from build123d import *

# Parameters (mm, degrees)
SKETCH1_W               = 48
SKETCH1_H               = 45
BOSS_EXTRUDE1_DEPTH     = 3
BOSS_EXTRUDE2_DEPTH     = 37
SKETCH3_W               = 3
SKETCH3_H               = 40
BOSS_EXTRUDE3_DEPTH     = 30
BOSS_EXTRUDE4_DEPTH     = 3
FILLET1_R               = 10
FILLET2_R               = 5
CHAMFER1_SIZE           = 2
SKETCH5_R               = 1.75
SKETCH5_R_2             = 12.5
CUT_EXTRUDE1_DEPTH      = 91.65064234
RIB2_REACH              = 82.792
SKETCH6_WALL_W          = 183.583291708
SKETCH6_WALL_H          = 5
LPATTERN2_COUNT         = 2
LPATTERN2_PITCH         = 15
MIRROR1_COPY_1_REACH    = 82.792
MIRROR1_COPY_1_SKETCH_W = 183.583291708
MIRROR1_COPY_1_SKETCH_H = 5
SKETCH7_R               = 1.75
CUT_EXTRUDE2_DEPTH      = 97.982157929


with BuildPart() as part:
    # Sketch1 → Boss-Extrude1 (new body)
    with BuildSketch(Plane(origin=(0, 0, 0), x_dir=(1, 0, 0), z_dir=(0, 1, 0))):
        with Locations((0, -1.5)):
            Rectangle(SKETCH1_W, SKETCH1_H)
    extrude(amount=BOSS_EXTRUDE1_DEPTH)

    # Sketch2 → Boss-Extrude2 (add)
    with BuildSketch(Plane.XZ):
        Polygon((-21, 21), (21, 21), (21, -21), (24, -21), (24, 24), (-24, 24), (-24, -21), (-21, -21), align=None)
    extrude(amount=BOSS_EXTRUDE2_DEPTH)

    # Sketch3 → Boss-Extrude3 (add)
    with BuildSketch(Plane(origin=(24, 0, 0), x_dir=(0, 0, -1), z_dir=(1, 0, 0))):
        with Locations((19.5, -17)):
            Rectangle(SKETCH3_W, SKETCH3_H)
    extrude(amount=BOSS_EXTRUDE3_DEPTH)

    # Sketch4 → Boss-Extrude4 (add)
    with BuildSketch(Plane(origin=(0, 0, -21), x_dir=(-1, 0, 0), z_dir=(0, 0, -1))):
        Polygon((24, 3), (65.213203436, -38.213203436), (45.213203436, -58.213203436), (24, -37), align=None)
    extrude(amount=-BOSS_EXTRUDE4_DEPTH)

    # Fillet1
    fillet1_edges = [part.edges().sort_by_distance(p)[0] for p in [
        (24, -17, -18),
        (-24, -17, -18),
    ]]
    fillet(fillet1_edges, radius=FILLET1_R)

    # Fillet2
    fillet2_edges = [part.edges().sort_by_distance(p)[0] for p in [
        (21, -18.5, -21),
        (-21, -18.5, -21),
    ]]
    fillet(fillet2_edges, radius=FILLET2_R)

    # Chamfer1
    chamfer1_edges = [part.edges().sort_by_distance(p)[0] for p in [
        (24, -17, 24),
        (-24, -17, 24),
    ]]
    chamfer(chamfer1_edges, length=CHAMFER1_SIZE)

    # Sketch5 → Cut-Extrude1 (cut, through all)
    with BuildSketch(Plane.XZ):
        with Locations(Location((-15.5, 15.5, 0), (0, 0, 270))):
            Circle(SKETCH5_R)
        with Locations(Location((15.5, 15.5, 0), (0, 0, 270))):
            Circle(SKETCH5_R)
        with Locations(Location((15.5, -15.5, 0), (0, 0, 270))):
            Circle(SKETCH5_R)
        with Locations(Location((-15.5, -15.5, 0), (0, 0, 270))):
            Circle(SKETCH5_R)
        with Locations(Location((0, 0, 0), (0, 0, 270))):
            Circle(SKETCH5_R_2)
    extrude(amount=-CUT_EXTRUDE1_DEPTH, mode=Mode.SUBTRACT)

    # Sketch6 wall → Rib2 (add, up to next)
    with BuildSketch(Plane(origin=(-31.071067812, -17, -10.928932188), x_dir=(-0.707106781187, 0, -0.707106781187), z_dir=(-0.707106781187, 0, 0.707106781187)), mode=Mode.PRIVATE) as rib2_sk1:
        Rectangle(SKETCH6_WALL_W, SKETCH6_WALL_H)
    rib2_tool1 = extrude(rib2_sk1.sketch, amount=-RIB2_REACH, mode=Mode.PRIVATE) - part.part
    rib2 = rib2_tool1.solids().sort_by_distance((-31.071067812, -17, -10.928932188))[0]
    add(rib2)

    # LPattern2: Rib2 ×2
    with Locations(*[(0, -i * LPATTERN2_PITCH, 0) for i in range(1, LPATTERN2_COUNT)]):
        add(rib2)

    # Mirror1: Rib2 across plane
    add(rib2.mirror(Plane(origin=(0, 0, 0), x_dir=(0, 0, 1), z_dir=(1, 0, 0))))

    # Mirror1 copy 1 sketch → Mirror1 copy 1 (add, up to next)
    with BuildSketch(Plane(origin=(31.071067812, -32, -10.928932188), x_dir=(0.707106781187, 0, -0.707106781187), z_dir=(0.707106781187, 0, 0.707106781187)), mode=Mode.PRIVATE) as mirror1_copy_1_sk1:
        Rectangle(MIRROR1_COPY_1_SKETCH_W, MIRROR1_COPY_1_SKETCH_H)
    mirror1_copy_1_tool1 = extrude(mirror1_copy_1_sk1.sketch, amount=-MIRROR1_COPY_1_REACH, mode=Mode.PRIVATE) - part.part
    add(mirror1_copy_1_tool1.solids().sort_by_distance((31.071067812, -32, -10.928932188))[0])

    # Sketch7 → Cut-Extrude2 (cut, through all)
    with BuildSketch(Plane.XY.offset(-18)):
        with Locations((44, -7)):
            Circle(SKETCH7_R)
        with Locations((44, -27)):
            Circle(SKETCH7_R)
        with Locations((-50.338834765, -37.480970389)):
            Circle(SKETCH7_R)
    extrude(amount=-CUT_EXTRUDE2_DEPTH, mode=Mode.SUBTRACT)


solid = part.part
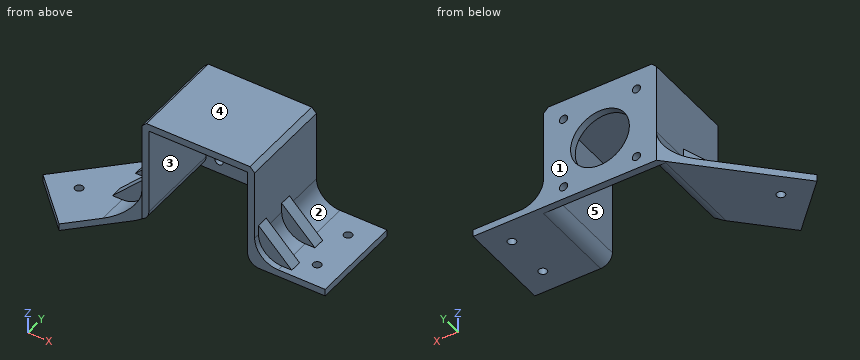
Can you work these out from the model? Positions are in its coordinate system, mm. Face numbers are marked on the shaded views. A direction names the side the tool comes from. Round coordinates to 2 decimals unless told otherwise and drop trailing zeros. Order: outer loops, then holes, each group sorted by start corner. A loop starts at its lowest first (then second) coordinate and runs counter-clockwise, first axis right, second up. Notation, with made-up numbers: (7.5, 6.5) - (17.5, 6.5) arc R21 cw to (17.5, 25.5) - close; hole circle Ø3 at (16, 18). An arc over 180 degrees is marked (long way). Answer in a Markdown table with one row per item.
(1) Please list where these lines run through material, in increasing order: L1, parallel to Z at x = 15, y = 1; L2, parallel to X at y = 2, z = -15; L3, parallel to X at y = -36.5, z = -7. Write a range as from..to.
From the geometry:
| item | result |
|---|---|
| L1 | z = -21..-17.18, -13.82..13.82, 17.18..24 |
| L2 | x = -25..-17.18, -13.82..13.82, 17.18..26.86 |
| L3 | x = -24..-21, 21..24 |
(2) Suppose I cut it at D-D, the plane z = 11. Please give me the cut outline in (x, y).
From the geometry:
| item | result |
|---|---|
| outline | (-24, -37) - (-21, -37) - (-21, 0) - (-5.94, 0) - (-5.94, 3) - (-24, 3) - close; (5.94, 0) - (21, 0) - (21, -37) - (24, -37) - (24, 3) - (5.94, 3) - close |
(3) Suppose I cut it at C-C, the plane y = -13. Please give me the cut outline in (x, z), plus the area to 3 significant figures.
From the geometry:
| item | result |
|---|---|
| outline | (-40, -21) - (-26, -21) arc R5 ccw to (-21, -16) - (-21, 21) - (21, 21) - (21, -16) arc R5 ccw to (26, -21) - (54, -21) - (54, -18) - (34, -18) arc R10 cw to (24, -8) - (24, 22) - (22, 24) - (-22, 24) - (-24, 22) - (-24, -8) arc R10 cw to (-34, -18) - (-40, -18) - close |
| area | 562 mm2 |
(4) If we mould it in two halves opening along X, with no side actions, what happens to the marked faces 1, 2 and 3? For each: released by +X, released by -X, zero draft, split by the parting line, or undercut.
From the geometry:
| item | result |
|---|---|
| face 1 | zero draft |
| face 2 | released by +X |
| face 3 | undercut |
(5) Suppose I cut it at B-B, the plane x = 15.5. Please give me the cut outline in (y, z).
From the geometry:
| item | result |
|---|---|
| outline | (-37, 21) - (0, 21) - (0, 17.25) - (3, 17.25) - (3, 24) - (-37, 24) - close; (0, -21) - (3, -21) - (3, -17.25) - (0, -17.25) - close; (0, -13.75) - (3, -13.75) - (3, 13.75) - (0, 13.75) - close |
(6) Which directions (+Z, -Z, +X, -X, +Y, -Y) give clear straight access to the entire face, cutting with the end or side of a thin tool? Please do the marked faces 4 and 5.
From the geometry:
| item | result |
|---|---|
| face 4 | +Z, +X, -X, +Y, -Y |
| face 5 | -Z, -Y |
(7) Suppose I cut it at A-A, the plane z = 0. Please give me the cut outline in (x, y), plus the area to 3 significant figures.
From the geometry:
| item | result |
|---|---|
| outline | (-24, -37) - (-21, -37) - (-21, 0) - (-12.5, 0) - (-12.5, 3) - (-24, 3) - close; (12.5, 0) - (21, 0) - (21, -37) - (24, -37) - (24, 3) - (12.5, 3) - close |
| area | 291 mm2 |
(8) For P1, Ø1.5, axis at x = -13.5, z = 10.5, coming from the -Y side; P2, Ø4, axis at x = 31, z = -13.5, coming from the -Y side; P3, Ø9.5, axis at x = -52.5, y = -38.5, coming from the +Z side; P4, Ø12, axis at x = -44.5, z = -11.5, coming from the +Y side, each with a flat end and sliding along its axis, tell me the tip position at first contact or that it passes through.
From the geometry:
| item | result |
|---|---|
| P1 | stops at y = 0 |
| P2 | stops at y = -34.5 |
| P3 | stops at z = -18 |
| P4 | passes through |
